Design review of the part built by this model. Coordinates are the model's own, in mm. A direction names the side the tool comes from. Coordinates: 2 decimals unless noted, no trailing zeros. Loops run counter-clockwise (first coordinate to the right, second up) from the corner with the lowest first, then second, coordinate; pieces in that order, holes last. Notation, with made-up numbers: (-16, -38) -> (32, -38) arc R13 ccw to (32, -16) -> close; hole circle Ø9 at (76, 25.25). An arc over 180 degrees is marked (long way). Use CSV: the item, a comma, the result in double quotes.
```python
from build123d import *

# Parameters (mm, degrees)
SKETCH1_W           = 15.2
SKETCH1_H           = 15.88
BOSS_EXTRUDE1_DEPTH = 16.38
CUT_EXTRUDE1_DEPTH  = 15.38
SKETCH3_W           = 1.25
SKETCH3_H           = 1.5
BOSS_EXTRUDE2_DEPTH = 6


with BuildPart() as part:
    # Sketch1 → Boss-Extrude1 (new body)
    with BuildSketch(Plane.XY):
        Rectangle(SKETCH1_W, SKETCH1_H)
    extrude(amount=BOSS_EXTRUDE1_DEPTH)

    # Sketch2 → Cut-Extrude1 (cut)
    with BuildSketch(Plane.XY.offset(16.38)):
        Polygon((-2, 6.74), (2, 6.74), (2, 4.74), (2.75, 4.74), (2.75, 2.74), (5.9, 2.74), (5.9, 0.74), (6.6, 0.74), (6.6, -3.44), (5.9, -3.44), (5.9, -5.44), (-5.9, -5.44), (-5.9, -3.44), (-6.6, -3.44), (-6.6, 0.74), (-5.9, 0.74), (-5.9, 2.74), (-2.75, 2.74), (-2.75, 4.74), (-2, 4.74), align=None)
    extrude(amount=-CUT_EXTRUDE1_DEPTH, mode=Mode.SUBTRACT)

    # Sketch3 → Boss-Extrude2 (add, symmetric)
    with BuildSketch(Plane(origin=(0, 0, 0), x_dir=(1, 0, 0), z_dir=(0, 1, 0))):
        with Locations((8.225, -14.13)):
            Rectangle(SKETCH3_W, SKETCH3_H)
        with Locations((-8.225, -14.13)):
            Rectangle(SKETCH3_W, SKETCH3_H)
    extrude(amount=BOSS_EXTRUDE2_DEPTH, both=True)


solid = part.part
```
Item 1: Add section A-A (z = 9.75). Give the boundary of the cut face in (x, y).
Checked values:
outline,"(-7.6, -7.94) -> (7.6, -7.94) -> (7.6, 7.94) -> (-7.6, 7.94) -> close; hole (-6.6, -3.44) -> (-5.9, -3.44) -> (-5.9, -5.44) -> (5.9, -5.44) -> (5.9, -3.44) -> (6.6, -3.44) -> (6.6, 0.74) -> (5.9, 0.74) -> (5.9, 2.74) -> (2.75, 2.74) -> (2.75, 4.74) -> (2, 4.74) -> (2, 6.74) -> (-2, 6.74) -> (-2, 4.74) -> (-2.75, 4.74) -> (-2.75, 2.74) -> (-5.9, 2.74) -> (-5.9, 0.74) -> (-6.6, 0.74) -> close"
Item 2: Add section C-C (x = 4.5). Give the boundary of the cut face in (y, z).
Checked values:
outline,"(-7.94, 0) -> (7.94, 0) -> (7.94, 16.38) -> (2.74, 16.38) -> (2.74, 1) -> (-5.44, 1) -> (-5.44, 16.38) -> (-7.94, 16.38) -> close"
Item 3: To check wall thickness, follow line 1 along X through (y, z) = (5, 7); line 2 along Y through (x, z) = (3.75, 5.5); line 3 along X through (y, z) = (1, 6.75). State the ranges of each line that lie inside material, in increasing order.
Checked values:
line 1,"-7.6 to -2, 2 to 7.6"
line 2,"-7.94 to -5.44, 2.74 to 7.94"
line 3,"-7.6 to -5.9, 5.9 to 7.6"
Item 4: Draft analysis for pull direction Y (two halves, no side actions). For faces 1 (the face through (0, 7.94, 8)), 2 (the face through (8, -6, 14)), 3 (the face through (0, -1, 1)), state which applies: pulls with the +Y half, pulls with the -Y half, needs draft (parallel to the pull), parting line crosses it, or undercut.
Checked values:
face 1,"pulls with the +Y half"
face 2,"pulls with the -Y half"
face 3,"undercut"
Item 5: Machinability: for faces 4 (the face through (-8, 6, 14)), 5 (the face through (-8, 0, 14.88)), 6 (the face through (5.9, 2, 9)), 7 (the face through (8, 6, 14)), 8 (the face through (-8, 0, 13.38)), which of the approach directions +Z, -Z, +X, -X, +Y, -Y give a long, thin tool a straight path to every point of the face, cutting with its end or side? Answer none if there is none.
Checked values:
face 4,"+Z, -Z, -X, +Y"
face 5,"+Z, -X, +Y, -Y"
face 6,"+Z"
face 7,"+Z, -Z, +X, +Y"
face 8,"-Z, -X, +Y, -Y"
Item 6: Add section D-D (y = -0.5). Give the boundary of the cut face in (x, z), then the cut area to 3 significant figures.
Checked values:
outline,"(-8.85, 13.38) -> (-7.6, 13.38) -> (-7.6, 0) -> (7.6, 0) -> (7.6, 13.38) -> (8.85, 13.38) -> (8.85, 14.88) -> (7.6, 14.88) -> (7.6, 16.38) -> (6.6, 16.38) -> (6.6, 1) -> (-6.6, 1) -> (-6.6, 16.38) -> (-7.6, 16.38) -> (-7.6, 14.88) -> (-8.85, 14.88) -> close"
area,"49.7 mm^2"
Item 7: Clearance check with flat-ended pins moving along their axes: pin 1 (3.5 mm diameter, centred on y = -1, z = 6, fed in from -X); pin 2 (1.4 mm diameter, centred on x = 8, y = -1, fed in from +Z); pin 3 (3.5 mm diameter, centred on y = -0.5, z = 9, fed in from +X). State where each tip first meets the part, or that it passes through.
Checked values:
pin 1,"x = -7.6"
pin 2,"z = 16.38"
pin 3,"x = 7.6"
Item 8: Add section B-B (y = 3.25). Give the boundary of the cut face in (x, z), then the cut area to 3 significant figures.
Checked values:
outline,"(-8.85, 13.38) -> (-7.6, 13.38) -> (-7.6, 0) -> (7.6, 0) -> (7.6, 13.38) -> (8.85, 13.38) -> (8.85, 14.88) -> (7.6, 14.88) -> (7.6, 16.38) -> (2.75, 16.38) -> (2.75, 1) -> (-2.75, 1) -> (-2.75, 16.38) -> (-7.6, 16.38) -> (-7.6, 14.88) -> (-8.85, 14.88) -> close"
area,"168 mm^2"
